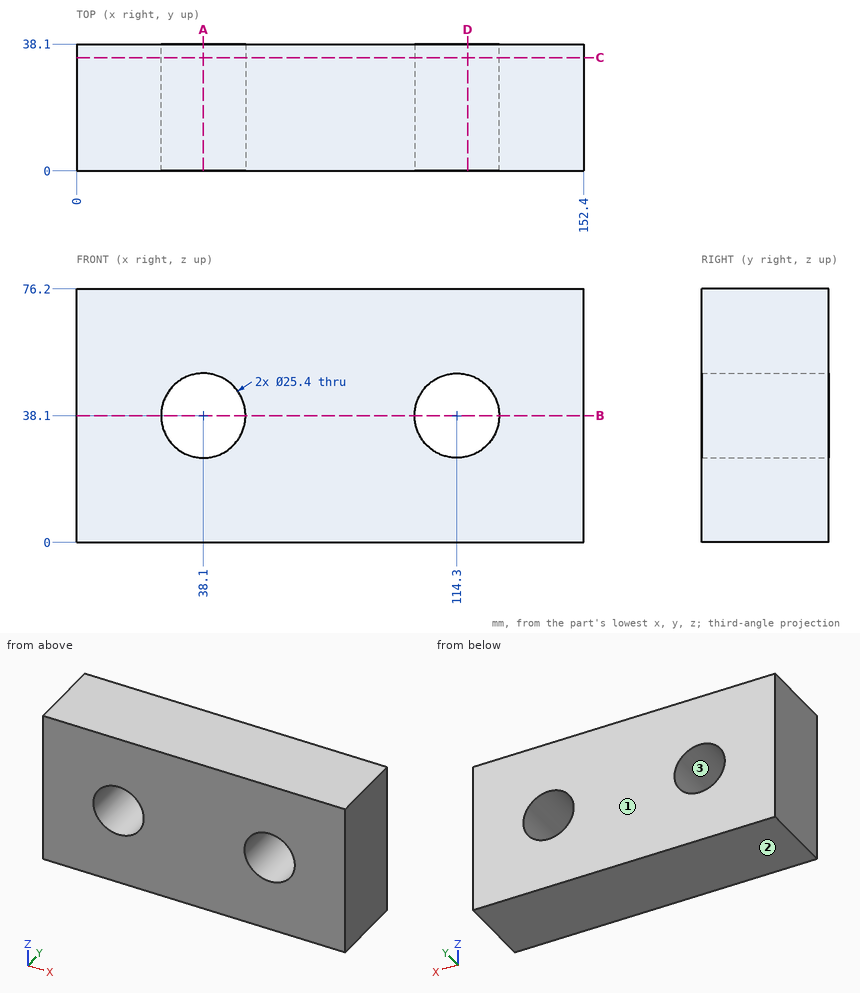
For this review, use the dimensioned drawing (mm, ordinates from the lowest corner) and the shaded views. Give positions to 0.01 mm unless a question says otherwise; leave off trailing zeros. Write each loop counter-clockwise with the first axis right and the second up, starting at its lowest first coordinate (ties: lowest second). Pieces come first, ordered by that corner, then holes.
(1) Consider section D-D, the plane x = 117.5. Give the boundary of the cut face in (y, z), and give its area (3 significant figures).
(2) To check wall thickness, follow L1, parallel to X at y = 21, z = 38; L2, parallel to X at y = 33, z = 44; L3, parallel to Z at x = 38.1, y = 30. State the ranges of each line that lie inside material, in increasing order.
(3) Consider section A-A, the plane x = 38.1. Give the boundary of the cut face in (y, z).
(4) Consider section B-B, the plane z = 38.1. Give the boundary of the cut face in (x, y).
(5) Consider section C-C, the plane y = 34. Give the boundary of the cut face in (x, z), and give its area (3 significant figures).
(6) The part is to be moulded in two halves that separate along Z. For the marked faces 1, 2 and 3, say which applies: released by +Z, released by -Z, zero draft, split by the parting line, or undercut.
Returned:
1. outline: (0, 0) - (38.1, 0) - (38.1, 25.81) - (0, 25.81) - close; (0, 50.39) - (38.1, 50.39) - (38.1, 76.2) - (0, 76.2) - close
1. area: 1,970 mm2
2. L1: x = 0 to 25.4, 50.8 to 101.6, 127 to 152.4
2. L2: x = 0 to 26.85, 49.35 to 103.05, 125.55 to 152.4
2. L3: z = 0 to 25.4, 50.8 to 76.2
3. outline: (0, 0) - (38.1, 0) - (38.1, 25.4) - (0, 25.4) - close; (0, 50.8) - (38.1, 50.8) - (38.1, 76.2) - (0, 76.2) - close
4. outline: (0, 0) - (25.4, 0) - (25.4, 38.1) - (0, 38.1) - close; (50.8, 0) - (101.6, 0) - (101.6, 38.1) - (50.8, 38.1) - close; (127, 0) - (152.4, 0) - (152.4, 38.1) - (127, 38.1) - close
5. outline: (0, 0) - (152.4, 0) - (152.4, 76.2) - (0, 76.2) - close; hole circle Ø25.4 at (38.1, 38.1); hole circle Ø25.4 at (114.3, 38.1)
5. area: 10,600 mm2
6. face 1: zero draft
6. face 2: released by -Z
6. face 3: undercut
